Can you work these out from the drawing? Everything is in mm from the part's minimum corner. A direction names the side the tool comes from. Round coordinates to 2 decimals unless told otherwise and drop trailing zeros. Loops run counter-clockwise (first coordinate to the right, second up) from the corner with the lowest first, then second, coordinate; pieces in that order, holes last. Notation, with made-up numbers: (-8, -28) -> (9, -28) arc R15 ccw to (9, -19) -> close; hole circle Ø1 at (11, 60.25). An arc over 180 degrees is marked (long way). One line per item, written item: value.
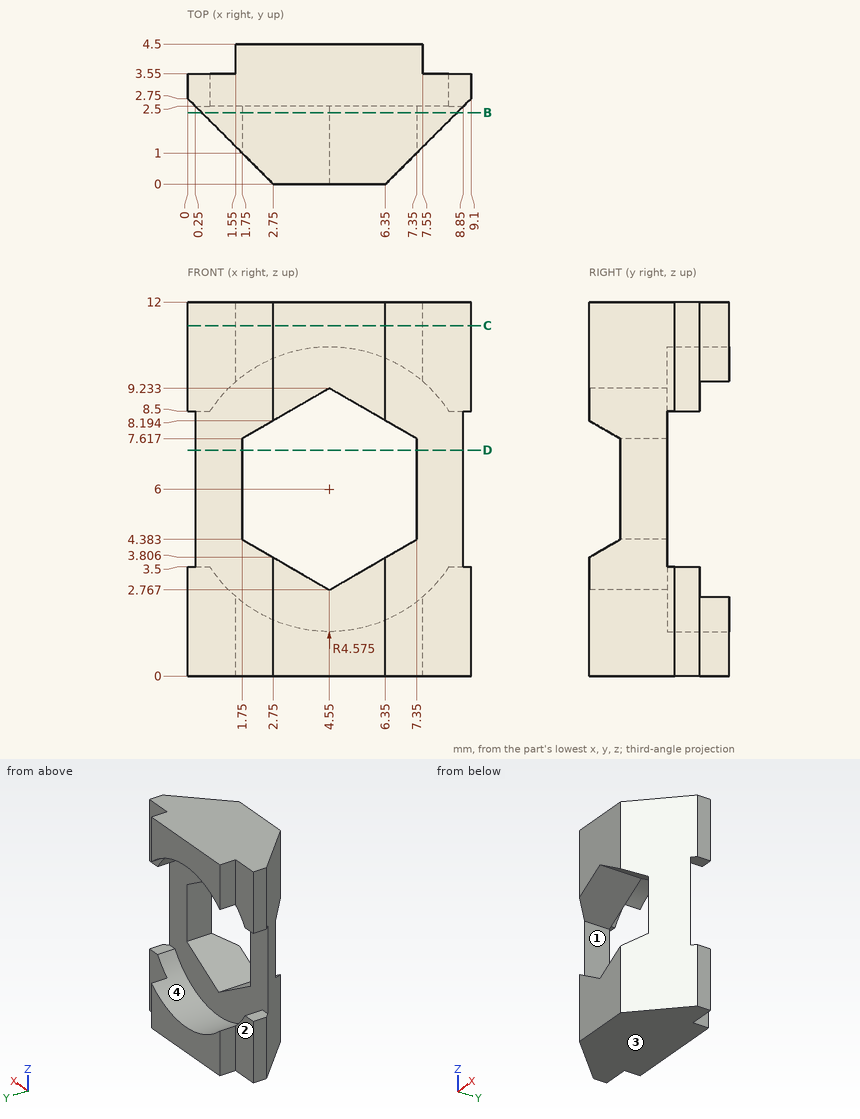
(1) If I drill on L1, parallel to Z at x = 0.5, y = 2.8; L2, parallel to Y at x = 3, z = 3.5; L3, parallel to Z at x = 4.75, y = 3.35, over which ranges is the centre line in solid material (lowest first)?
Recorded:
L1: 0 to 3.5, 8.5 to 12
L2: 0 to 2.5
L3: 0 to 1.43, 10.57 to 12
(2) If we section it at C-C, the plane z = 11.25: Please give me the cut outline in (x, y).
Recorded:
outline: (0, 2.75) -> (2.75, 0) -> (6.35, 0) -> (9.1, 2.75) -> (9.1, 3.55) -> (7.55, 3.55) -> (7.55, 4.5) -> (1.55, 4.5) -> (1.55, 3.55) -> (0, 3.55) -> close
(3) If we section it at B-B, the plane y = 2.3: Please give me the cut outline in (x, z).
Recorded:
outline: (0.45, 0) -> (8.65, 0) -> (8.65, 12) -> (0.45, 12) -> close; hole (1.75, 4.38) -> (4.55, 2.77) -> (7.35, 4.38) -> (7.35, 7.62) -> (4.55, 9.23) -> (1.75, 7.62) -> close
(4) If we section it at D-D, the plane z = 7.25: Please give me the cut outline in (x, y).
Recorded:
outline: (0.25, 2.5) -> (1.75, 1) -> (1.75, 2.5) -> close; (7.35, 1) -> (8.85, 2.5) -> (7.35, 2.5) -> close
(5) I'm going to push flat-ended pins straight in: pin 1 Ø0.8 at (y, z) = (2, 5.5) entering from -X; pin 2 Ø2 at (x, z) = (1.5, 4) entering from +Y; pin 3 Ø0.5 at (y, z) = (2, 6) entering from +X. Where does each tip first touch, or does it pass through?
Recorded:
pin 1: x = 0.35
pin 2: y = 3.55
pin 3: x = 8.6
(6) For the marked faces 1, 2, 3 and 4, which set-ups out of +Z, -Z, +X, -X, +Y, -Y let a thin tool reach every point of the face, with its end or its side?
Recorded:
face 1: +Y, -Y
face 2: +Z, -Z, -X, +Y
face 3: -Z, +X, -X, +Y, -Y
face 4: +Y
